Could you check a few things on this model? Use its own coordinates, in mm. Face numbers are marked on the shaded views. A direction names the side the tool comes from. Coordinates: 2 decimals unless noted, no trailing zeros. Order: outer loops, then holes, each group sorted by start corner. A loop starts at its lowest first (then second) coordinate and runs counter-clockwise, first axis right, second up. Notation, with made-up numbers: (-27.5, 50.5) - (22.5, 50.5) arc R12 ccw to (22.5, 65.5) - close; hole circle Ø10 at (-8, -38.75). An arc over 180 degrees is marked (long way). Answer as a JSON object with one key per item and string values. Group by question number.
(1) Will these pins go through, and if not, where does the flat tip stop? P1, Ø6.5, axis at x = 12, y = 0, coming from the +Z side; P2, Ø1.8, axis at x = -13.5, y = 1, coming from the +Z side.
(2) Please list where these lines run through material, in increasing order: probe 1 along Y at (x, z) = (-12.5, 3.2); probe 2 along Y at (x, z) = (-12.5, 1.1); probe 3 along X at (y, z) = (0, 0.9).
(3) Imagine slicing it at A-A, the plane y = 12.5. Write out the boundary of the cut face in (x, z), and give its area (4 significant figures).
(4) We'd pull the mould along X, two halves only. Please class the marked faces 3, 4 and 5: pulls with the +X half, pulls with the -X half, needs draft (parallel to the pull), parting line crosses it, or undercut.
(5) Imagine slicing it at B-B, the plane z = 0.95. Write out the boundary of the cut face in (x, y), and give its area (3 significant figures).
(6) Which directions (+Z, -Z, +X, -X, +Y, -Y) give clear straight access to the entire face, cutting with the end or side of a thin tool? Please do the marked faces 1 and 2.
(7) Imagine slicing it at C-C, the plane x = -12.5. Write out the boundary of the cut face in (y, z), and give its area (4 significant figures).
(8) Imagine slicing it at D-D, the plane z = 2.9. Write out the boundary of the cut face in (x, y), and give its area (3 significant figures).
from build123d import *

# Parameters (mm, degrees)
F0_W     = 35
F0_H     = 35
F0_R     = 1.5
F0_R_2   = 2
F1_DEPTH = 5
F2_R     = 3
F3_DEPTH = 3.5
F4_SIZE  = 1
F5_SIZE  = 0.49999


# Not quite as in the source:
# - a fillet or chamfer is up to 0.001 mm smaller than in the source, because OpenCascade refuses the exact size


with BuildPart() as f1:
    # F0 (on Top) → F1 (new body)
    with BuildSketch(Plane.XY):
        Rectangle(F0_W, F0_H)
        with Locations((-12.5, -12.5)):
            Circle(F0_R, mode=Mode.SUBTRACT)
        with Locations((12.5, -12.5)):
            Circle(F0_R, mode=Mode.SUBTRACT)
        with Locations((-12.5, 0)):
            Circle(F0_R_2, mode=Mode.SUBTRACT)
        with Locations((-12.5, 12.5)):
            Circle(F0_R, mode=Mode.SUBTRACT)
        with Locations((12.5, 0)):
            Circle(F0_R_2, mode=Mode.SUBTRACT)
        with Locations((12.5, 12.5)):
            Circle(F0_R, mode=Mode.SUBTRACT)
    extrude(amount=F1_DEPTH)

    # F2 (on face) → F3 (cut)
    with BuildSketch(Plane.XY.offset(5)):
        with Locations((-12.5, 0)):
            Circle(F2_R)
        with Locations((12.5, 0)):
            Circle(F2_R)
    extrude(amount=-F3_DEPTH, mode=Mode.SUBTRACT)

    # F4
    f4_edges = [f1.edges().sort_by_distance(p)[0] for p in [
        (-17.5, -17.5, 2.5),
        (-17.5, 17.5, 2.5),
        (17.5, -17.5, 2.5),
        (17.5, 17.5, 2.5),
    ]]
    chamfer(f4_edges, length=F4_SIZE)

    # F5 (size 0.5 in the source; OpenCascade refuses exactly that, so slightly less here)
    f5_edges = [f1.edges().sort_by_distance(p)[0] for p in [
        (17.5, 0, 5),
        (0, 17.5, 5),
        (-17.5, 0, 5),
        (17.5, 0, 0),
        (0, -17.5, 5),
        (0, -17.5, 0),
        (0, 17.5, 0),
        (-17.5, 0, 0),
    ]]
    chamfer(f5_edges, length=F5_SIZE)


solid = f1.part
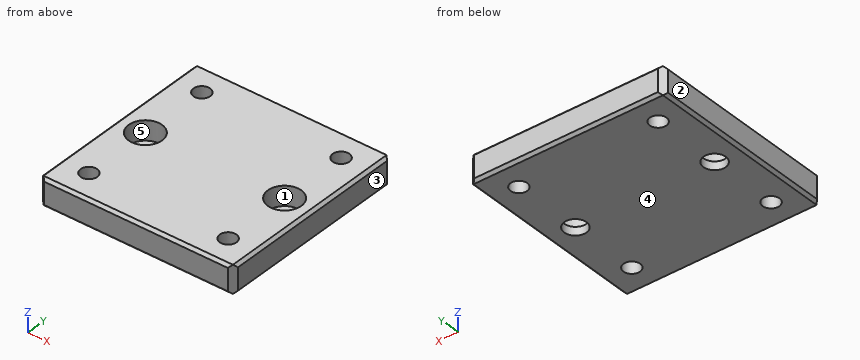
Result set:
{
 "1": {"P1": "stops at z = 5", "P2": "stops at z = 1.5"},
 "2": {"probe 1": "y = -17.5 to -14, -11 to -3, 3 to 11, 14 to 17.5", "probe 2": "y = -17.5 to -14, -11 to -2, 2 to 11, 14 to 17.5", "probe 3": "x = -17.5 to -14.5, -10.5 to 10.5, 14.5 to 17.5"},
 "3": {"outline": "(-17.5, 0.5) - (-17, 0) - (-14, 0) - (-14, 5) - (-17, 5) - (-17.5, 4.5) - close; (-11, 0) - (11, 0) - (11, 5) - (-11, 5) - close; (14, 0) - (17, 0) - (17.5, 0.5) - (17.5, 4.5) - (17, 5) - (14, 5) - close", "area": "144.5 mm^2"},
 "4": {"face 3": "pulls with the +X half", "face 4": "needs draft", "face 5": "undercut"},
 "5": {"outline": "(-17.5, -16.5) - (-16.5, -17.5) - (16.5, -17.5) - (17.5, -16.5) - (17.5, 16.5) - (16.5, 17.5) - (-16.5, 17.5) - (-17.5, 16.5) - close; hole circle Ø4 at (-12.5, 0); hole circle Ø3 at (-12.5, -12.5); hole circle Ø3 at (-12.5, 12.5); hole circle Ø4 at (12.5, 0); hole circle Ø3 at (12.5, -12.5); hole circle Ø3 at (12.5, 12.5)", "area": "1,170 mm^2"},
 "6": {"face 1": "+Z", "face 2": "+Z, -Z, -X, +Y, -Y"},
 "7": {"outline": "(-17.5, 0.5) - (-17, 0) - (-14, 0) - (-14, 5) - (-17, 5) - (-17.5, 4.5) - close; (-11, 0) - (-2, 0) - (-2, 1.5) - (-3, 1.5) - (-3, 5) - (-11, 5) - close; (2, 0) - (11, 0) - (11, 5) - (3, 5) - (3, 1.5) - (2, 1.5) - close; (14, 0) - (17, 0) - (17.5, 0.5) - (17.5, 4.5) - (17, 5) - (14, 5) - close", "area": "117.5 mm^2"},
 "8": {"outline": "(-17.5, -16.5) - (-16.5, -17.5) - (16.5, -17.5) - (17.5, -16.5) - (17.5, 16.5) - (16.5, 17.5) - (-16.5, 17.5) - (-17.5, 16.5) - close; hole circle Ø6 at (-12.5, 0); hole circle Ø3 at (-12.5, -12.5); hole circle Ø3 at (-12.5, 12.5); hole circle Ø6 at (12.5, 0); hole circle Ø3 at (12.5, -12.5); hole circle Ø3 at (12.5, 12.5)", "area": "1,140 mm^2"}
}
